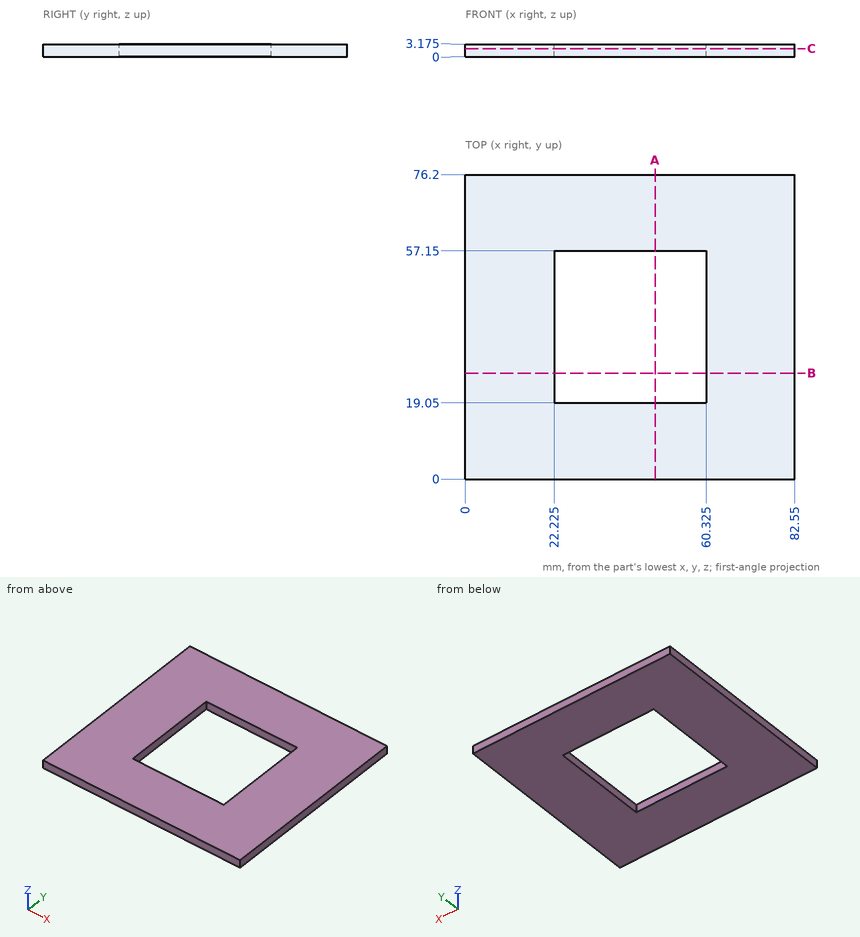
Input: dimensioned drawing with shaded views. Units: mm. Origin: part minimum x, y, z. Coordinates: 2 decimals unless noted, no trailing zeros. Order: outer loops, then holes, each group sorted by start corner. A loop starts at its lowest first (then second) coordinate and runs counter-clockwise, first axis right, second up. Notation, with made-up numbers: (34.25, 33.25) - (84.25, 33.25) arc R29 cw to (84.25, 55.25) - close; hole circle Ø3 at (17, 78.5). An arc over 180 degrees is marked (long way). Put each result on its own line as item: value.
1. Cut plane B-B on y = 26.5. Return the cut outline in (x, z) (3 decimals), then the cut area to 3 significant figures.
Report:
outline: (0, 0) - (22.225, 0) - (22.225, 3.175) - (0, 3.175) - close; (60.325, 0) - (82.55, 0) - (82.55, 3.175) - (60.325, 3.175) - close
area: 141 mm2
2. Cut plane C-C on z = 2. Return the cut outline in (x, y) (3 decimals).
Report:
outline: (0, 0) - (82.55, 0) - (82.55, 76.2) - (0, 76.2) - close; hole (22.225, 19.05) - (60.325, 19.05) - (60.325, 57.15) - (22.225, 57.15) - close
3. Cut plane A-A on x = 47.5. Return the cut outline in (y, z) (3 decimals).
Report:
outline: (0, 0) - (19.05, 0) - (19.05, 3.175) - (0, 3.175) - close; (57.15, 0) - (76.2, 0) - (76.2, 3.175) - (57.15, 3.175) - close
4. Line query: line 1 along Y through (x, z) = (55, 0.45); line 2 along X through (y, z) = (41, 1.15) (3 decimals). Output: solid intervals per line, ascending.
Report:
line 1: y = 0 to 19.05, 57.15 to 76.2
line 2: x = 0 to 22.225, 60.325 to 82.55
5. Contact query for a flat-ended pin moving along its axis: pin 1 Ø2 at (x, y) = (66.5, 39.5) entering from -Z. Output: stop coordinate, or through.
Report:
pin 1: stops at z = 0
